Here's the drawing with two shaded views (mm, measured from the low corner). I have some questions. A direction names the side the tool comes from. Coordinates: 2 decimals unless noted, no trailing zeros. Loops run counter-clockwise (first coordinate to the right, second up) from the corner with the lowest first, then second, coordinate; pieces in that order, holes last.
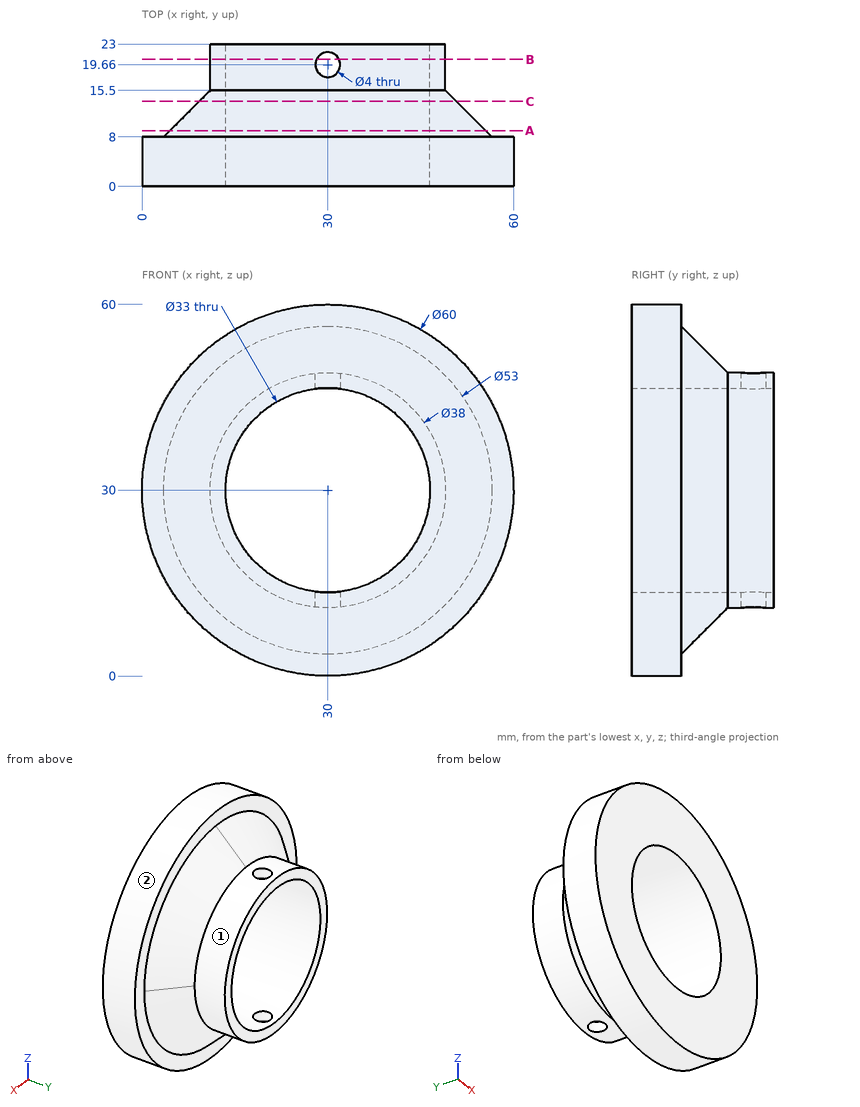
(1) I'm going to push flat-ended pins straight in: pin 1 (1 mm diameter, centred on x = 28, y = 19.5, fed in from +Z); pin 2 (3 mm diameter, centred on y = 4.5, z = 35.5, fed in from +X); pin 3 (1.5 mm diameter, centred on x = 10.5, z = 48.5, fed in from +Y); pin 4 (5 mm diameter, centred on x = 15, z = 31.5, fed in from +Y). Where does each tip first touch, or does it pass through?
Check values:
pin 1: stops at z = 48.91
pin 2: stops at x = 59.73
pin 3: stops at y = 8.37
pin 4: stops at y = 23
(2) I want a section at C-C on y = 13.75. Write out the boundary of the cut face in (x, z).
Check values:
outline: circle Ø41.5 at (30, 30); hole circle Ø33 at (30, 30)
(3) Which directions (+Z, -Z, +X, -X, +Y, -Y) give clear straight access to the entire face, cutting with the end or side of a thin tool? Please do the marked faces 1 and 2.
Check values:
face 1: +Y
face 2: +Y, -Y
(4) I want a section at B-B on y = 20.5. Write out the boundary of the cut face in (x, z) (1 decimal).
Check values:
outline: (28.2, 11.1) - (28.2, 13.6) arc R16.5 cw to (28.2, 46.4) - (28.2, 48.9) arc R19 ccw to start; (31.8, 11.1) arc R19 ccw to (31.8, 48.9) - (31.8, 46.4) arc R16.5 cw to (31.8, 13.6) - close
(5) If I drill on probe 1 along Y at (x, z) = (30, 47.15); probe 2 along X at (y, z) = (18, 30); probe 3 along X at (y, z) = (20, 37) (1 decimal), over which ranges is the centre line in solid material (lowest first)?
Check values:
probe 1: y = 0 to 17.66, 21.66 to 23
probe 2: x = 11 to 13.5, 46.5 to 49
probe 3: x = 12.3 to 15.1, 44.9 to 47.7
(6) I want a section at A-A on y = 9. Write out the boundary of the cut face in (x, z), then the cut area to 3 significant figures.
Check values:
outline: circle Ø51 at (30, 30); hole circle Ø33 at (30, 30)
area: 1,190 mm2
